CAD build for the part. Positions are in the model's coordinates, mm. Give positions to 0.01 mm unless a question says otherwise; leave off trailing zeros. Order: outer loops, then holes, each group sorted by start corner. A loop starts at its lowest first (then second) coordinate and runs counter-clockwise, first axis right, second up.
from build123d import *

# Parameters (mm, degrees)
F0_R     = 1
F1_DEPTH = 1.25
F2_R     = 3


with BuildPart() as f1:
    # F0 (on Top) → F1 (new body)
    with BuildSketch(Plane.XY):
        Polygon((0, 17.3524001093), (0, 42.3524001093), (-74, 42.3524001093), (-74, 17.3524001093), (-67.080681713, 0.2000030523), (-6.919318287, 0.2000030523), align=None)
        with Locations((-65.375, 1.8524001093)):
            Circle(F0_R, mode=Mode.SUBTRACT)
        with Locations((-8.625, 1.8524001093)):
            Circle(F0_R, mode=Mode.SUBTRACT)
        with Locations((-71.3, 40.3524001093)):
            Circle(F0_R, mode=Mode.SUBTRACT)
        with Locations((-2.7, 40.3524001093)):
            Circle(F0_R, mode=Mode.SUBTRACT)
    extrude(amount=F1_DEPTH)

    # F2
    f2_edges = [f1.edges().sort_by_distance(p)[0] for p in [
        (0, 42.3524, 0.625),
        (-74, 42.3524, 0.625),
        (-74, 17.3524, 0.625),
        (0, 17.3524, 0.625),
        (-6.919318, 0.200003, 0.625),
        (-67.080682, 0.200003, 0.625),
    ]]
    fillet(f2_edges, radius=F2_R)


solid = f1.part
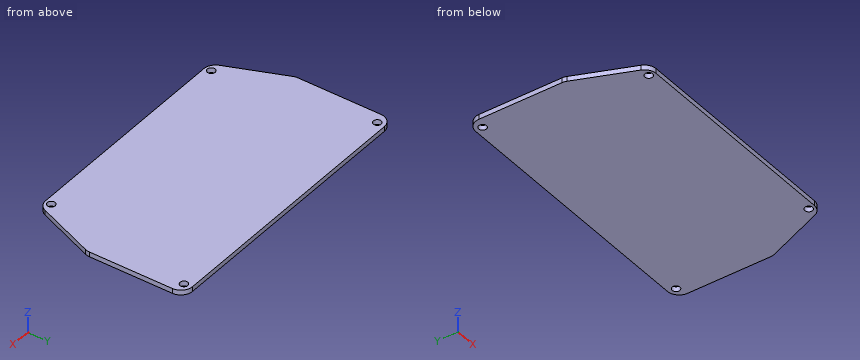
1. Pin check, flat tip, straight feed: P1, Ø2.5, axis at x = -8.62, y = 1.85, coming from the +Z side. Stop position of the tip, or through.
2. Saw through at B-B on y = 6.5. Give the cut face in (x, z).
3. Wall check: line 1 (Y direction, x = -2.7, z = 0.9); line 2 (X direction, y = 13, z = 0.8); line 3 (X direction, y = 17, z = 0.8). Give the ranges that are in metal, low to high.
4. Saw through at A-A on z = 1.05. Give the cut face in (x, y) (3 decimals), plus the area to 3 significant figures.
Reported:
1. P1: stops at z = 1.25
2. outline: (-69.62, 0) - (-4.38, 0) - (-4.38, 1.25) - (-69.62, 1.25) - close
3. line 1: y = 10.66 to 39.35, 41.35 to 42.34
3. line 2: x = -72.24 to -1.76
3. line 3: x = -73.85 to -0.15
4. outline: (-74, 17.935) arc R3 ccw to (-73.782, 16.812) - (-67.838, 2.078) arc R3 ccw to (-65.056, 0.2) - (-8.944, 0.2) arc R3 ccw to (-6.162, 2.078) - (-0.218, 16.812) arc R3 ccw to (0, 17.935) - (0, 39.352) arc R3 ccw to (-3, 42.352) - (-71, 42.352) arc R3 ccw to (-74, 39.352) - close; hole circle Ø2 at (-71.3, 40.352); hole circle Ø2 at (-65.375, 1.852); hole circle Ø2 at (-8.625, 1.852); hole circle Ø2 at (-2.7, 40.352)
4. area: 2,980 mm2
